from build123d import *

# Parameters (mm, degrees)
SKETCH_1_W      = 100
SKETCH_1_H      = 120
SKETCH_1_R      = 1.5
SKETCH_1_W_2    = 20
SKETCH_1_H_2    = 45
EXTRUDE_1_DEPTH = 3
FILLET_1_R      = 3
FILLET_2_R      = 2


with BuildPart() as part:
    # 草图1 → 凸台-拉伸1 (new body)
    with BuildSketch(Plane(origin=(0, 0, 0), x_dir=(1, 0, 0), z_dir=(0, 1, 0))):
        Rectangle(SKETCH_1_W, SKETCH_1_H)
        with Locations(Location((-45, -50, 0), (0, 0, 270))):
            Circle(SKETCH_1_R, mode=Mode.SUBTRACT)
        with Locations(Location((-45, -30, 0), (0, 0, 270))):
            Circle(SKETCH_1_R, mode=Mode.SUBTRACT)
        Polygon((-35.320508076, -15), (-18, -25), (-18, -45), (-35.320508076, -55), align=None, mode=Mode.SUBTRACT)
        with Locations(Location((-45, -10, 0), (0, 0, 270))):
            Circle(SKETCH_1_R, mode=Mode.SUBTRACT)
        Polygon((-35.320508076, -10), (-35.320508076, 10), (-18, 20), (-18, -20), align=None, mode=Mode.SUBTRACT)
        with Locations((0, -27.5)):
            Rectangle(SKETCH_1_W_2, SKETCH_1_H_2, mode=Mode.SUBTRACT)
        with Locations((0, 27.5)):
            Rectangle(SKETCH_1_W_2, SKETCH_1_H_2, mode=Mode.SUBTRACT)
        with Locations(Location((45, -50, 0), (0, 0, 270))):
            Circle(SKETCH_1_R, mode=Mode.SUBTRACT)
        Polygon((18, -25), (35.320508076, -15), (35.320508076, -55), (18, -45), align=None, mode=Mode.SUBTRACT)
        with Locations(Location((45, -30, 0), (0, 0, 270))):
            Circle(SKETCH_1_R, mode=Mode.SUBTRACT)
        Polygon((35.320508076, -10), (18, -20), (18, 20), (35.320508076, 10), align=None, mode=Mode.SUBTRACT)
        with Locations(Location((45, -10, 0), (0, 0, 270))):
            Circle(SKETCH_1_R, mode=Mode.SUBTRACT)
        with Locations(Location((-45, 10, 0), (0, 0, 270))):
            Circle(SKETCH_1_R, mode=Mode.SUBTRACT)
        with Locations(Location((-45, 30, 0), (0, 0, 270))):
            Circle(SKETCH_1_R, mode=Mode.SUBTRACT)
        Polygon((-35.320508076, 15), (-35.320508076, 55), (-18, 45), (-18, 25), align=None, mode=Mode.SUBTRACT)
        with Locations(Location((-45, 50, 0), (0, 0, 270))):
            Circle(SKETCH_1_R, mode=Mode.SUBTRACT)
        with Locations(Location((45, 10, 0), (0, 0, 270))):
            Circle(SKETCH_1_R, mode=Mode.SUBTRACT)
        with Locations(Location((45, 30, 0), (0, 0, 270))):
            Circle(SKETCH_1_R, mode=Mode.SUBTRACT)
        Polygon((35.320508076, 15), (18, 25), (18, 45), (35.320508076, 55), align=None, mode=Mode.SUBTRACT)
        with Locations(Location((45, 50, 0), (0, 0, 270))):
            Circle(SKETCH_1_R, mode=Mode.SUBTRACT)
    extrude(amount=EXTRUDE_1_DEPTH)

    # 圆角1
    fillet_1_edges = [part.edges().sort_by_distance(p)[0] for p in [
        (-50, 1.5, 60),
        (-50, 1.5, -60),
        (50, 1.5, -60),
        (50, 1.5, 60),
    ]]
    fillet(fillet_1_edges, radius=FILLET_1_R)

    # 圆角2
    fillet_2_edges = [part.edges().sort_by_distance(p)[0] for p in [
        (18, 1.5, -25),
        (35.320508076, 1.5, -15),
        (35.320508076, 1.5, -55),
        (18, 1.5, -45),
        (18, 1.5, 20),
        (35.320508076, 1.5, 10),
        (35.320508076, 1.5, -10),
        (18, 1.5, -20),
        (-18, 1.5, 25),
        (-35.320508076, 1.5, 15),
        (-35.320508076, 1.5, 55),
        (-18, 1.5, 45),
        (-35.320508076, 1.5, -55),
        (-35.320508076, 1.5, -15),
        (-18, 1.5, -25),
        (-18, 1.5, -45),
        (-35.320508076, 1.5, -10),
        (-35.320508076, 1.5, 10),
        (-18, 1.5, 20),
        (-18, 1.5, -20),
        (18, 1.5, 45),
        (35.320508076, 1.5, 55),
        (35.320508076, 1.5, 15),
        (18, 1.5, 25),
        (10, 1.5, 5),
        (-10, 1.5, 5),
        (-10, 1.5, 50),
        (10, 1.5, 50),
        (10, 1.5, -50),
        (-10, 1.5, -50),
        (-10, 1.5, -5),
        (10, 1.5, -5),
    ]]
    fillet(fillet_2_edges, radius=FILLET_2_R)


solid = part.part
Check sheet for the modelled part. Datum: model origin and axes. Units: mm. Give positions to 0.01 mm unless a question says otherwise; leave off trailing zeros. Write each loop counter-clockwise with the first axis right and the second up, starting at its lowest first coordinate (ties: lowest second). Pieces come first, ordered by that corner, then holes. Notation, with made-up numbers: (-26, -35.5) -> (-3, -35.5) arc R17 cw to (-3, -14.5) -> close; hole circle Ø4 at (77.5, -11.5). An arc over 180 degrees is marked (long way). Write item = value, one per line.
Item 1: Sectioned sample at A-A on x = 45. Record the boundary of the cut face in (y, z).
Output:
outline = (0, -60) -> (3, -60) -> (3, -51.5) -> (0, -51.5) -> close; (0, -48.5) -> (3, -48.5) -> (3, -31.5) -> (0, -31.5) -> close; (0, -28.5) -> (3, -28.5) -> (3, -11.5) -> (0, -11.5) -> close; (0, -8.5) -> (3, -8.5) -> (3, 8.5) -> (0, 8.5) -> close; (0, 11.5) -> (3, 11.5) -> (3, 28.5) -> (0, 28.5) -> close; (0, 31.5) -> (3, 31.5) -> (3, 48.5) -> (0, 48.5) -> close; (0, 51.5) -> (3, 51.5) -> (3, 60) -> (0, 60) -> close
Item 2: Gauge pin test, flat end, axial feed: pin 1 (3.5 mm diameter, centred on x = 45, z = 10, fed in from +Y). Record the tip position at first contact, or that the pin passes through.
Output:
pin_1 = 3
Item 3: Sectioned sample at B-B on z = -34. Record the boundary of the cut face in (x, y), and give its area (3 significant figures).
Output:
outline = (-50, 0) -> (-35.32, 0) -> (-35.32, 3) -> (-50, 3) -> close; (-18, 0) -> (-10, 0) -> (-10, 3) -> (-18, 3) -> close; (10, 0) -> (18, 0) -> (18, 3) -> (10, 3) -> close; (35.32, 0) -> (50, 0) -> (50, 3) -> (35.32, 3) -> close
area = 136 mm^2
Item 4: Sectioned sample at C-C on x = -6.5. Record the boundary of the cut face in (y, z).
Output:
outline = (0, -60) -> (3, -60) -> (3, -50) -> (0, -50) -> close; (0, -5) -> (3, -5) -> (3, 5) -> (0, 5) -> close; (0, 50) -> (3, 50) -> (3, 60) -> (0, 60) -> close
Item 5: Scan lines: probe 1 along Z at (x, y) = (-6, 1.75); probe 2 along X at (y, z) = (0.95, -36.5); probe 3 along X at (y, z) = (2.1, -30). Record each from-to range of solid material in increasing order. Write a range as from..to.
Output:
probe_1 = -60..-50, -5..5, 50..60
probe_2 = -50..-35.32, -18..-10, 10..18, 35.32..50
probe_3 = -50..-46.5, -43.5..-35.32, -18..-10, 10..18, 35.32..43.5, 46.5..50
Item 6: Sectioned sample at D-D on y = 1.95. Count the separate pieces of the cut face and the enclosed holes in it, and give its area (3 significant figures).
Output:
separate_pieces = 1
enclosed_holes = 20
area = 7,030 mm^2
Item 7: Release check for a two-part mould opening along Z. For faces 1 (the flat face through (0, 1, 50)), 2 (the flat face through (-50, 1, 1)), 3 (the flat face through (-18, 1, -35)) record: +Z half, -Z half, draft (parallel to the pull), parting line (faces both ways), or undercut.
Output:
face_1 = undercut
face_2 = draft
face_3 = undercut
